from build123d import *

# Parameters (mm, degrees)
BOSS_EXTRUDE1_DEPTH = 5
FILLET1_R           = 5
SKETCH3_R           = 2.3
BOSS_EXTRUDE2_DEPTH = 5


with BuildPart() as part:
    # Lid → Boss-Extrude1 (new body)
    with BuildSketch(Plane(origin=(0, 0, 0), x_dir=(1, 0, 0), z_dir=(0, 1, 0))):
        Polygon((-80, -175), (80, -175), (80, 30), (80, 32.01), (78.04, 36.53), (65, 50), (-65, 50), (-78.04, 36.53), (-80, 32.01), (-80, 30), align=None)
    extrude(amount=BOSS_EXTRUDE1_DEPTH)

    # Fillet1
    fillet1_edges = [part.edges().sort_by_distance(p)[0] for p in [
        (0, 5, 175),
        (-79.02, 5, -34.27),
        (-80, 5, 71.495),
        (-71.52, 5, -43.265),
        (0, 5, -50),
        (71.52, 5, -43.265),
        (79.02, 5, -34.27),
        (80, 5, 71.495),
    ]]
    fillet(fillet1_edges, radius=FILLET1_R - 0.0001)  # a hair under: the kernel refuses the full size

    # Sketch3 → Boss-Extrude2 (add)
    with BuildSketch(Plane(origin=(0, 0, 0), x_dir=(1, 0, 0), z_dir=(0, 1, 0))):
        with Locations(Location((-62.5, 40, 0), (0, 0, 270))):
            Circle(SKETCH3_R)
        with Locations(Location((62.5, 40, 0), (0, 0, 270))):
            Circle(SKETCH3_R)
        with Locations(Location((75, -170, 0), (0, 0, 270))):
            Circle(SKETCH3_R)
        with Locations(Location((-75, -170, 0), (0, 0, 270))):
            Circle(SKETCH3_R)
        Polygon((-77.4, -57.7), (-77.4, -62.3), (-75.1, -62.3), (-75.1, -60), (-75.1, -57.7), align=None)
        Polygon((75.1, -57.7), (77.4, -57.7), (77.4, -62.3), (75.1, -62.3), (75.1, -60), align=None)
    extrude(amount=-BOSS_EXTRUDE2_DEPTH)


solid = part.part
Verification items for the finished model (mm, model axes). A direction names the side the tool comes from. Give positions to 0.01 mm unless a question says otherwise; leave off trailing zeros. Order: outer loops, then holes, each group sorted by start corner. A loop starts at its lowest first (then second) coordinate and runs counter-clockwise, first axis right, second up. Notation, with made-up numbers: M 87.25,88 L 93.25,88 A26 cw 93.25,111 Z; hole C -6.75,11 d1. An arc over 180 degrees is marked long. Use one line per item in the form item = value. Start each with the question number.
Q1. Mould release check, pull along Z, two halves, no side actions. Record for faces 1 (the flat face through (75.1, -2, 60)), 2 (the cylindrical face through (72.755, -2.465, 169.501)), 3 (the cylindrical face through (60.255, -2.465, -40.499)): +Z half, -Z half, draft (parallel to the pull), parting line (faces both ways), or undercut.
Q2. Scan lines: line 1 along X through (y, z) = (0.5, 90); line 2 along X through (y, z) = (4, -30); line 3 along Z through (x, y) = (13, 0.25). Record each from-to range of solid material in increasing order. Write a range as [from, to].
Q3. Go/stop test with flat-tipped pins: pin 1 Ø1 at (x, y) = (49, 1) entering from -Z; pin 2 Ø2 at (x, y) = (41.5, 3) entering from -Z; pin 3 Ø1.2 at (x, y) = (76, -3.5) entering from -Z. Record where each tip stops, or that it passes through.
Q4. Section check A-A (y = -3). Enter the section's corners in (x, z), then the cut area to 3 significant figures.
Q5. Access from +Z, -Z, +X, -X, +Y, -Y to the whole of each face (thin tool, end or side, straight path). Record for faces 4 (the cylindrical face through (-64.745, -2.465, -40.499)), 5 (the flat face through (77.4, -2, 60)), 6 (the flat face through (-75.1, -2, 60)).
Evaluation:
q1.face_1 = draft
q1.face_2 = undercut
q1.face_3 = parting line
q2.line_1 = [-79.97, 79.97]
q2.line_2 = [-78, 78]
q2.line_3 = [-49.99, 174.99]
q3.pin_1 = -49.97
q3.pin_2 = -49.58
q3.pin_3 = 57.7
q4.outline = M -77.4,57.7 L -75.1,57.7 L -75.1,62.3 L -77.4,62.3 Z; C -75,170 d4.6; C -62.5,-40 d4.6; C 62.5,-40 d4.6; C 75,170 d4.6; M 75.1,57.7 L 77.4,57.7 L 77.4,62.3 L 75.1,62.3 Z
q4.area = 87.6 mm2
q5.face_4 = -Y
q5.face_5 = +Z, -Z, +X, -Y
q5.face_6 = -Z, -Y
